```python
from build123d import *

# Parameters (mm, degrees)
AXIAL_BLANK_PROFILE_W                          = 5
AXIAL_BLANK_PROFILE_H                          = 41
TWO_START                                      = -22
TWO_FITTING_ROUTE_CLEARANCE_BORES_DI_2_R       = 8.25
TWO_FITTING_ROUTE_CLEARANCE_BORES_DIAMET_DEPTH = 5
THREE_START                                    = -22
THREE_LONG_MOUNTING_SCREW_CLEARANCES_SKE_R     = 1.7
THREE_LONG_MOUNTING_SCREW_CLEARANCES_DEPTH     = 5
THREE_START_2                                  = -20
THREE_M2_LOCATOR_RECEIVING_PILOTS_DE_2_R       = 0.8
THREE_M2_LOCATOR_RECEIVING_PILOTS_DEPTH3_DEPTH = 3


with BuildPart() as part:
    # Axial blank profile → Native revolved blank (revolve)
    with BuildSketch(Plane.XY, mode=Mode.PRIVATE) as native_revolved_blank_sk:
        with Locations((-19.5, 20.5)):
            Rectangle(AXIAL_BLANK_PROFILE_W, AXIAL_BLANK_PROFILE_H)
    revolve(native_revolved_blank_sk.sketch.rotate(Axis((-60, 0, 0), (1, 0, 0)), 90), axis=Axis((-60, 0, 0), (1, 0, 0)))

    # Two fitting-route clearance bores di 2 → Two fitting-route clearance bores diamet (cut)
    with BuildSketch(Plane(origin=(0, 0, 0), x_dir=(0, 0, -1), z_dir=(1, 0, 0)).offset(TWO_START)):
        with Locations((-13, 22.516660498)):
            Circle(TWO_FITTING_ROUTE_CLEARANCE_BORES_DI_2_R)
        with Locations((13, 22.516660498)):
            Circle(TWO_FITTING_ROUTE_CLEARANCE_BORES_DI_2_R)
    extrude(amount=TWO_FITTING_ROUTE_CLEARANCE_BORES_DIAMET_DEPTH, mode=Mode.SUBTRACT)

    # Three long mounting screw clearances sketch → Three long mounting screw clearances (cut)
    with BuildSketch(Plane(origin=(0, 0, 0), x_dir=(0, 0, -1), z_dir=(1, 0, 0)).offset(THREE_START)):
        with Locations((0, 37)):
            Circle(THREE_LONG_MOUNTING_SCREW_CLEARANCES_SKE_R)
        with Locations((-32.04293994, -18.5)):
            Circle(THREE_LONG_MOUNTING_SCREW_CLEARANCES_SKE_R)
        with Locations((32.04293994, -18.5)):
            Circle(THREE_LONG_MOUNTING_SCREW_CLEARANCES_SKE_R)
    extrude(amount=THREE_LONG_MOUNTING_SCREW_CLEARANCES_DEPTH, mode=Mode.SUBTRACT)

    # Three M2 locator receiving pilots de 2 → Three M2 locator receiving pilots depth3 (cut)
    with BuildSketch(Plane(origin=(0, 0, 0), x_dir=(0, 0, -1), z_dir=(1, 0, 0)).offset(THREE_START_2)):
        with Locations((-24.248711306, 14)):
            Circle(THREE_M2_LOCATOR_RECEIVING_PILOTS_DE_2_R)
        with Locations((0, -28)):
            Circle(THREE_M2_LOCATOR_RECEIVING_PILOTS_DE_2_R)
        with Locations((24.248711306, 14)):
            Circle(THREE_M2_LOCATOR_RECEIVING_PILOTS_DE_2_R)
    extrude(amount=THREE_M2_LOCATOR_RECEIVING_PILOTS_DEPTH3_DEPTH, mode=Mode.SUBTRACT)


solid = part.part
```
Input: part model. Units: mm. Frame: model coordinates. Coordinates: 2 decimals unless noted, no trailing zeros. Write each loop counter-clockwise with the first axis right and the second up, starting at its lowest first coordinate (ties: lowest second). Pieces come first, ordered by that corner, then holes. Notation, with made-up numbers: (82.25, 81.25) -> (96.25, 81.25) arc R27 cw to (96.25, 112.25) -> close; hole circle Ø1 at (-7.5, -30). An arc over 180 degrees is marked (long way). Write each question's results on one line, items separated by ' | '.
Item 1: Section query C-C on y = -18.5. Return loops of the section in (x, z), plus the area to 3 significant figures.
Conclusion:
outline: (-22, -36.59) -> (-17, -36.59) -> (-17, -33.74) -> (-22, -33.74) -> close; (-22, -30.34) -> (-17, -30.34) -> (-17, 30.34) -> (-22, 30.34) -> close; (-22, 33.74) -> (-17, 33.74) -> (-17, 36.59) -> (-22, 36.59) -> close | area: 332 mm^2
Item 2: Section query A-A on y = 37. Return loops of the section in (x, z), plus the area to 3 significant figures.
Conclusion:
outline: (-22, -17.66) -> (-17, -17.66) -> (-17, -1.7) -> (-22, -1.7) -> close; (-22, 1.7) -> (-17, 1.7) -> (-17, 17.66) -> (-22, 17.66) -> close | area: 160 mm^2
Item 3: Pin query (flat end, axial travel): pin 1 Ø2 at (y, z) = (37, 0) entering from +X; pin 2 Ø0.5 at (y, z) = (14, -24.5) entering from +X. Return the tip coordinate at first contact, or that it passes through.
Conclusion:
pin 1: passes through | pin 2: stops at x = -20
Item 4: Section query D-D on x = -18.75. Count the separate pieces of the cut face and the enclosed holes in it, plus the area to 3 significant figures.
Conclusion:
separate pieces: 1 | enclosed holes: 8 | area: 4,820 mm^2
Item 5: Section query B-B on z = -8. Return loops of the section in (x, y), plus the area to 3 significant figures.
Conclusion:
outline: (-22, -40.21) -> (-17, -40.21) -> (-17, 15.95) -> (-22, 15.95) -> close; (-22, 29.08) -> (-17, 29.08) -> (-17, 40.21) -> (-22, 40.21) -> close | area: 336 mm^2
Item 6: Mould query, pull axis Y, two halves, no side actions, for faces 1 (the cylindrical face through (-19.465, 15.703, 37.874)), 2 (the cylindrical face through (-19.535, -17.989, -33.664)), 3 (the flat face through (-17, -1, 1)), 4 (the cylindrical face through (-19.54, 29.47, -17.44)). Classes: +Y half, -Y half, draft (parallel to the pull), parting line (faces both ways), or undercut.
Conclusion:
face 1: parting line | face 2: undercut | face 3: draft | face 4: undercut
Item 7: Material intervals for probe 1 along Y at (x, z) = (-20.15, 0); probe 2 along Z at (x, y) = (-20.8, 29.5); probe 3 along Y at (x, z) = (-19.1, -13), sorted ascending.
Conclusion:
probe 1: y = -41 to 35.3, 38.7 to 41 | probe 2: z = -28.47 to -17.39, -8.61 to 8.61, 17.39 to 28.47 | probe 3: y = -38.88 to 14.27, 30.77 to 38.88
